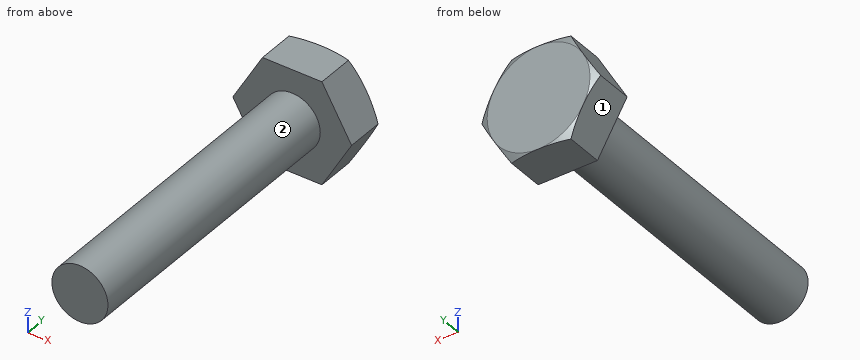
```python
from build123d import *

# Parameters (mm, degrees)
EXTRUDE_1_DEPTH = 2.2
SKETCH_3_R      = 1.5
EXTRUDE_2_DEPTH = 16


with BuildPart() as part:
    # 草图1 → 凸台-拉伸1 (new body)
    with BuildSketch(Plane(origin=(0, 0, 0), x_dir=(1, 0, 0), z_dir=(0, 1, 0))):
        Polygon((3.175426481, 0), (1.58771324, 2.75), (-1.58771324, 2.75), (-3.175426481, 0), (-1.58771324, -2.75), (1.58771324, -2.75), align=None)
    extrude(amount=EXTRUDE_1_DEPTH)

    # 草图2 → 切除-旋转1 (revolve, cut)
    with BuildSketch(Plane(origin=(0, 0, 0), x_dir=(0, 0, -1), z_dir=(1, 0, 0))):
        with BuildLine():
            Line((-2.75, 2.2), (-4.95, 2.2))
            Line((-4.95, 2.2), (-4.95, 0))
            ThreePointArc((-4.95, 0), (-4.068803604, 1.318803604), (-2.75, 2.2))
        make_face()
    revolve(axis=Axis((0, 0, 0), (0, 1, 0)), mode=Mode.SUBTRACT)

    # 草图3 → 凸台-拉伸2 (add)
    with BuildSketch(Plane.XZ):
        Circle(SKETCH_3_R)
    extrude(amount=EXTRUDE_2_DEPTH)


solid = part.part
```
Input: part model. Units: mm. Frame: model coordinates. Face numbers are marked on the shaded views. A direction names the side the tool comes from. Coordinates: 2 decimals unless noted, no trailing zeros. Write each loop counter-clockwise with the first axis right and the second up, starting at its lowest first coordinate (ties: lowest second). Pieces come first, ordered by that corner, then holes. Notation, with made-up numbers: (52.5, 16.25) -> (83.5, 16.25) arc R19 ccw to (83.5, 22.25) -> close; hole circle Ø3 at (-28.75, 16.5). An arc over 180 degrees is marked (long way). Answer as a JSON object with one key per item and string values.
1. Access query for the marked faces 1 and 2. Directions: +Z, -Z, +X, -X, +Y, -Y. A direction counts if a zero-diameter tool reaches every point of the face in a straight line with its end or side. Return the directions, or none.
Result set:
{"face 1": "-Z, -X, +Y, -Y", "face 2": "-Y"}
2. First-contact query: P1, Ø2, axis at x = 0, y = -1.5, coming from the +Z side. Flat tip, straight axial feed; report the tip coordinate or a pass-through.
Result set:
{"P1": "stops at z = 1.5"}
3. Material intervals for line 1 (Y direction, x = 1.5, z = 1.55); line 2 (X direction, y = -15, z = 0.1), sorted ascending. Write a range as from..to.
Result set:
{"line 1": "y = 0..2.2", "line 2": "x = -1.5..1.5"}
4. Section A-A on y = -4.25. Return the cut outline in (x, z), then the cut area to 3 significant figures.
Result set:
{"outline": "circle Ø3 at (0, 0)", "area": "7.07 mm2"}
